Can you work these out from the drawing? Everything is in mm from the part's minimum corner. A direction names the side the tool comes from. Round coordinates to 2 decimals unless told otherwise and drop trailing zeros. Order: outer loops, then holes, each group sorted by start corner. A loop starts at its lowest first (then second) coordinate and runs counter-clockwise, first axis right, second up. Notation, with made-up numbers: (50.25, 62) -> (81.25, 62) arc R23 cw to (81.25, 75) -> close; hole circle Ø5 at (17.25, 31.25). An arc over 180 degrees is marked (long way). Use a Markdown table: item, result. Add a question column.
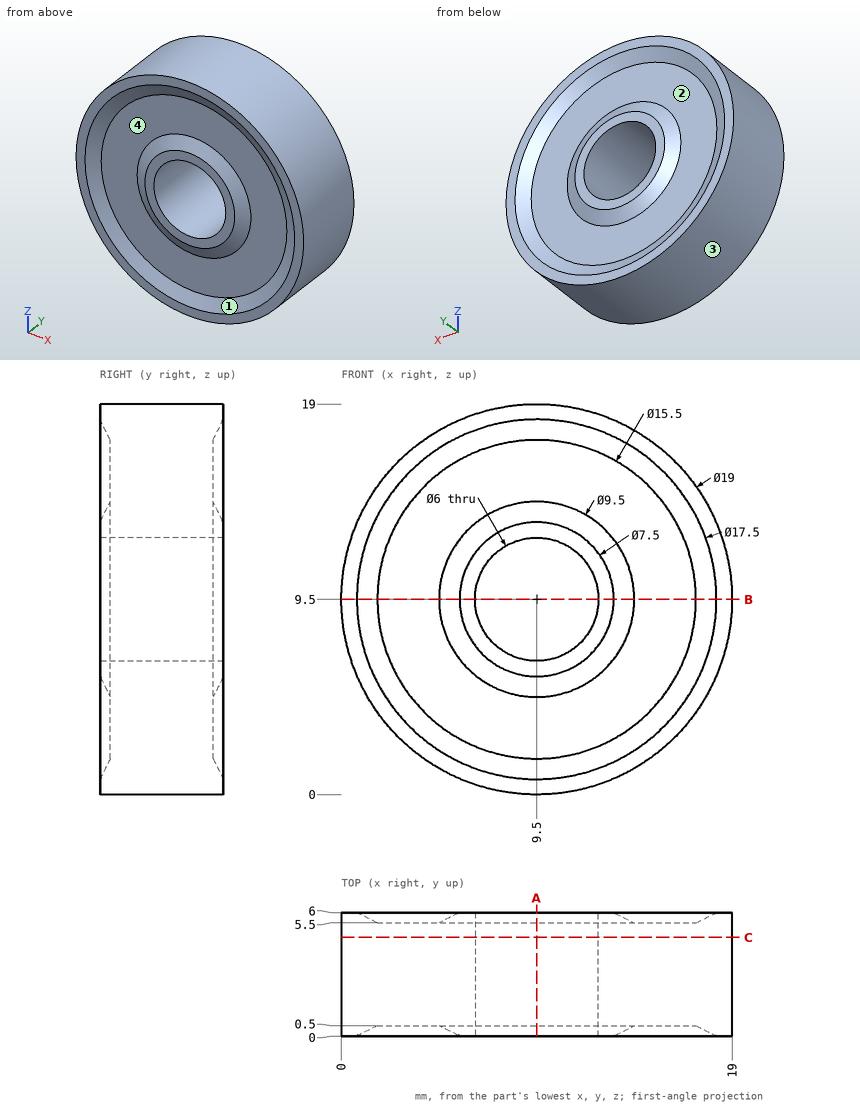
(1) I want a section at B-B on z = 9.5. List the corners of the cut face in (x, y) for me, and give its area (3 significant figures).
(2) If we mould it in two halves opening along X, with no side actions, what happens to the marked faces 3 and 4? For each: pulls with the +X half, pulls with the -X half, needs draft (parallel to the pull), parting line crosses it, or undercut.
(3) On a 3-axis mill with a long thin cutter (end or side, diameter ignored), from which of +Z, -Z, +X, -X, +Y, -Y can I reach the whole of each face in a straight line? I mean the marked faces 1 and 2. Say none if no direction works.
(4) Please list where these lines run through material, in increasing order: probe 1 along X at (y, z) = (2.25, 9.5); probe 2 along Y at (x, z) = (15.75, 11.5). Write a range as from..to.
(5) I'm going to push flat-ended pins straight in: P1, Ø1.5, axis at x = 2.5, y = 4.5, coming from the -Z side; P2, Ø1, axis at x = 10, y = 1.5, coming from the +Z side. Where does each tip first touch, or does it pass through?
(6) I want a section at A-A on x = 9.5. List the corners of the cut face in (y, z) for me, and give its area (3 significant figures).
(7) I want a section at C-C on y = 4.8. List the corners of the cut face in (x, z) for me, and give its area (3 significant figures).
Output:
| question | item | result |
|---|---|---|
| 1 | outline | (0, 0) -> (0.75, 0) -> (1.75, 0.5) -> (4.75, 0.5) -> (5.75, 0) -> (6.5, 0) -> (6.5, 6) -> (5.75, 6) -> (4.75, 5.5) -> (1.75, 5.5) -> (0.75, 6) -> (0, 6) -> close; (12.5, 0) -> (13.25, 0) -> (14.25, 0.5) -> (17.25, 0.5) -> (18.25, 0) -> (19, 0) -> (19, 6) -> (18.25, 6) -> (17.25, 5.5) -> (14.25, 5.5) -> (13.25, 6) -> (12.5, 6) -> close |
| 1 | area | 70.0 mm² |
| 2 | face 3 | parting line crosses it |
| 2 | face 4 | undercut |
| 3 | face 1 | -Y |
| 3 | face 2 | +Y |
| 4 | probe 1 | 0..6.5, 12.5..19 |
| 4 | probe 2 | 0.5..5.5 |
| 5 | P1 | z = 2.35 |
| 5 | P2 | z = 19 |
| 6 | outline | (0, 0) -> (6, 0) -> (6, 0.75) -> (5.5, 1.75) -> (5.5, 4.75) -> (6, 5.75) -> (6, 6.5) -> (0, 6.5) -> (0, 5.75) -> (0.5, 4.75) -> (0.5, 1.75) -> (0, 0.75) -> close; (0, 12.5) -> (6, 12.5) -> (6, 13.25) -> (5.5, 14.25) -> (5.5, 17.25) -> (6, 18.25) -> (6, 19) -> (0, 19) -> (0, 18.25) -> (0.5, 17.25) -> (0.5, 14.25) -> (0, 13.25) -> close |
| 6 | area | 70.0 mm² |
| 7 | outline | circle Ø19 at (9.5, 9.5); hole circle Ø6 at (9.5, 9.5) |
| 7 | area | 255 mm² |
